from build123d import *

# Parameters (mm, degrees)
F0_R     = 20.6375
F1_DEPTH = 1219.2
F3_R     = 20.6375
F4_DEPTH = 1270


with BuildPart() as f1:
    # F0 (on Front) → F1 (new body)
    with BuildSketch(Plane.XZ):
        Circle(F0_R)
    extrude(amount=F1_DEPTH)


with BuildPart() as f4:
    # F3 (on Right) → F4 (new body)
    with BuildSketch(Plane.YZ):
        Circle(F3_R)
    extrude(amount=F4_DEPTH)


solid = f4.part
Read the model definition and answer for the solid it produces. Units are mm, in the model's axes. Round coordinates to 2 decimals unless told otherwise and drop trailing zeros. Write each loop counter-clockwise with the first axis right and the second up, starting at its lowest first coordinate (ties: lowest second). Pieces come first, ordered by that corner, then holes.
1. The part is cut by section B-B, the plane y = -6.5. Determine the outline of the cut face in (x, z), then the cut area to 3 significant figures.
2. Given pin 1 Ø1 at (x, z) = (987, 8.5) entering from -Y; pin 2 Ø5 at (x, z) = (791, -15) entering from +Y; pin 3 Ø1 at (x, z) = (143.5, 15) entering from +Y, each flat-ended and moving along its own axis, determine where each tip first touches the part or whether it passes through.
3. The part is cut by section C-C, the plane z = -14. Determine the outline of the cut face in (x, y), then the cut area to 3 significant figures.
4. Straight lines are drawn through the part: L1, parallel to Y at x = 276.5, z = -1; L2, parallel to Y at x = 183, z = 2.5. For each, find the intervals that lie inside material, in ascending order.
5. The part is cut by section A-A, the plane x = 933. Determine the outline of the cut face in (y, z) (1 decimal), then the cut area to 3 significant figures.
Values:
1. outline: (0, -19.59) - (1270, -19.59) - (1270, 19.59) - (0, 19.59) - close
1. area: 49,800 mm2
2. pin 1: stops at y = -19.02
2. pin 2: stops at y = 16.42
2. pin 3: stops at y = 14.69
3. outline: (0, -15.16) - (1270, -15.16) - (1270, 15.16) - (0, 15.16) - close
3. area: 38,500 mm2
4. L1: y = -20.61 to 20.61
4. L2: y = -20.49 to 20.49
5. outline: circle Ø41.3 at (0, 0)
5. area: 1,340 mm2
